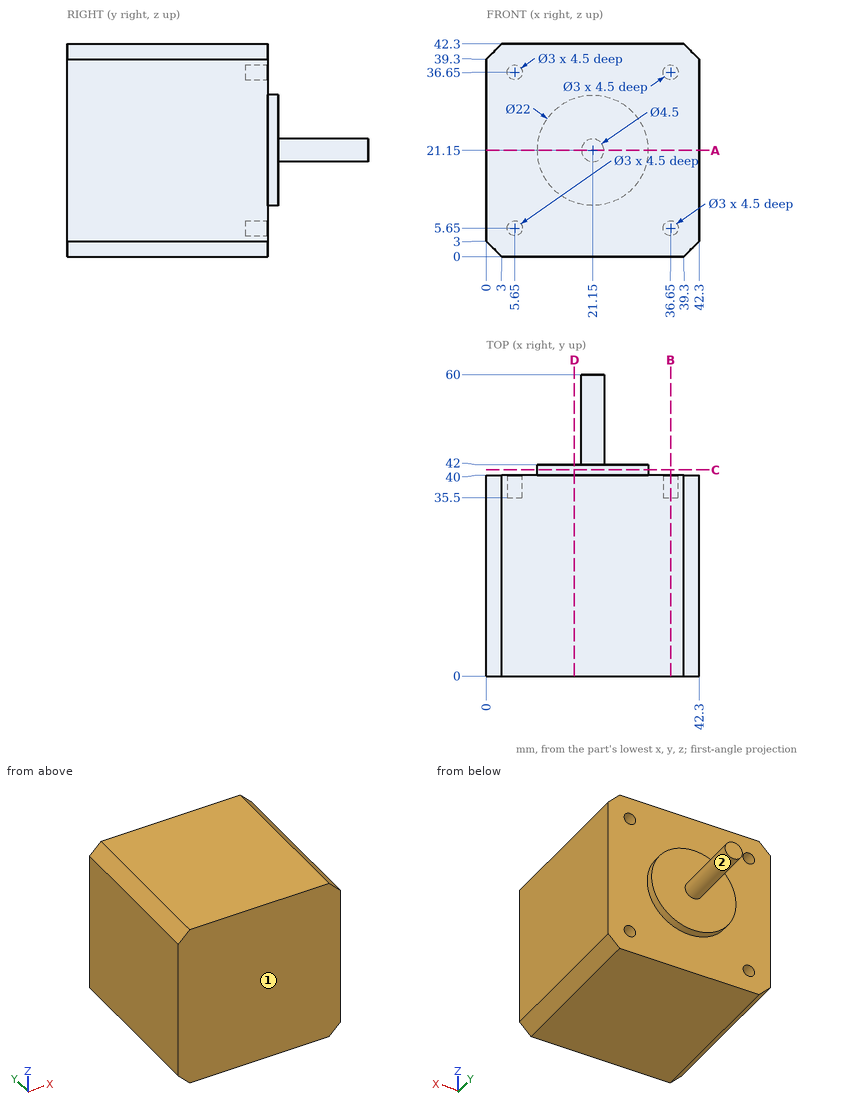
Here's the drawing with two shaded views (mm, measured from the low corner). I have some questions. A direction names the side the tool comes from. Coordinates: 2 decimals unless noted, no trailing zeros. Loops run counter-clockwise (first coordinate to the right, second up) from the corner with the lowest first, then second, coordinate; pieces in that order, holes last. Notation, with made-up numbers: (-37.75, 39) -> (17.25, 39) arc R22 ccw to (17.25, 58) -> close; hole circle Ø1 at (59.25, 16). An arc over 180 degrees is marked (long way). Answer in a Markdown table with one row per item.
(1) If I drill on probe 1 along Z at (x, y) = (36.65, 37.7); probe 2 along Z at (x, y) = (5, 36), over which ranges is the centre line in solid material (lowest first)?
Results found:
| item | result |
|---|---|
| probe 1 | z = 0 to 4.15, 7.15 to 35.15, 38.15 to 42.3 |
| probe 2 | z = 0 to 4.3, 7 to 35.3, 38 to 42.3 |
(2) Imagine slicing it at C-C (y = 41). List the corners of the cut face in (x, z) for me, plus the area to 3 significant figures.
Results found:
| item | result |
|---|---|
| outline | circle Ø22 at (21.15, 21.15) |
| area | 380 mm^2 |
(3) Imagine slicing it at D-D (x = 17.5). List the corners of the cut face in (y, z) for me, plus the area to 3 significant figures.
Results found:
| item | result |
|---|---|
| outline | (0, 0) -> (40, 0) -> (40, 10.77) -> (42, 10.77) -> (42, 31.53) -> (40, 31.53) -> (40, 42.3) -> (0, 42.3) -> close |
| area | 1,730 mm^2 |
(4) Will these pins go through, and if not, where does the flat tip stop? pin 1 Ø3.5 at (x, z) = (6, 5.5) entering from +Y; pin 2 Ø12 at (x, y) = (37, 51) entering from +Z; pin 3 Ø1.8 at (x, z) = (36.65, 5.65) entering from +Y; pin 4 Ø6 at (x, z) = (10, 14) entering from +Y.
Results found:
| item | result |
|---|---|
| pin 1 | stops at y = 40 |
| pin 2 | passes through |
| pin 3 | stops at y = 35.5 |
| pin 4 | stops at y = 42 |
(5) For the marked faces 1 and 2, which set-ups out of +Z, -Z, +X, -X, +Y, -Y let a thin tool reach every point of the face, with its end or its side?
Results found:
| item | result |
|---|---|
| face 1 | +Z, -Z, +X, -X, -Y |
| face 2 | +Y |
(6) Imagine slicing it at A-A (z = 21.15). List the corners of the cut face in (x, y) for me, plus the area to 3 significant figures.
Results found:
| item | result |
|---|---|
| outline | (0, 0) -> (42.3, 0) -> (42.3, 40) -> (32.15, 40) -> (32.15, 42) -> (23.4, 42) -> (23.4, 60) -> (18.9, 60) -> (18.9, 42) -> (10.15, 42) -> (10.15, 40) -> (0, 40) -> close |
| area | 1,820 mm^2 |
(7) Imagine slicing it at B-B (x = 36.65). List the corners of the cut face in (y, z) for me, plus the area to 4 significant figures.
Results found:
| item | result |
|---|---|
| outline | (0, 0) -> (40, 0) -> (40, 4.15) -> (35.5, 4.15) -> (35.5, 7.15) -> (40, 7.15) -> (40, 35.15) -> (35.5, 35.15) -> (35.5, 38.15) -> (40, 38.15) -> (40, 42.3) -> (0, 42.3) -> close |
| area | 1,665 mm^2 |
